from build123d import *

# Parameters (mm, degrees)
PAD_DEPTH = 1


with BuildPart() as part:
    # Sketch → Pad (new body)
    with BuildSketch(Plane.XY):
        with BuildLine():
            ThreePointArc((-1.225, 1.675), (-1.488415, 1.645732), (-1.73898, 1.559355))
            ThreePointArc((-4.225, 1), (-2.950915, 1.141565), (-1.73898, 1.559355))
            ThreePointArc((-4.225, 4), (-5.725, 2.5), (-4.225, 1))
            ThreePointArc((-4.225, 4), (-3.609451, 4.068394), (-3.023929, 4.270241))
            ThreePointArc((-1.225, 4.675), (-2.146951, 4.572561), (-3.023929, 4.270241))
            Line((-1.225, 4.675), (1.225012, 4.675))
            ThreePointArc((5.425, 0.475), (4.194853, 3.444844), (1.225012, 4.675))
            Line((5.425, -0.475), (5.425, 0.475))
            ThreePointArc((1.225, -4.675), (4.194848, -3.444848), (5.425, -0.475))
            Line((-1.225, -4.675), (1.225, -4.675))
            ThreePointArc((-3.023929, -4.270241), (-2.146951, -4.572561), (-1.225, -4.675))
            ThreePointArc((-3.023929, -4.270241), (-3.609451, -4.068394), (-4.225, -4))
            ThreePointArc((-4.225, -1), (-5.725, -2.5), (-4.225, -4))
            ThreePointArc((-1.73898, -1.559355), (-2.950915, -1.141565), (-4.225, -1))
            ThreePointArc((-1.73898, -1.559355), (-1.488415, -1.645732), (-1.225, -1.675))
            Line((-1.225, -1.675), (1.225, -1.675))
            ThreePointArc((1.225, -1.675), (2.073528, -1.323528), (2.425, -0.475))
            Line((2.425, 0.475), (2.425, -0.475))
            ThreePointArc((2.425, 0.475), (2.073532, 1.323524), (1.225012, 1.675))
            Line((-1.225, 1.675), (1.225012, 1.675))
        make_face()
    extrude(amount=PAD_DEPTH)


solid = part.part
Geometry check sheet. Reference: the model listing, model coordinates, mm. A direction names the side the tool comes from. Coordinates: 2 decimals unless noted, no trailing zeros. Order: outer loops, then holes, each group sorted by start corner. A loop starts at its lowest first (then second) coordinate and runs counter-clockwise, first axis right, second up. Notation, with made-up numbers: (54.25, -10) - (71.25, -10) arc R10 cw to (71.25, -5) - close; hole circle Ø8 at (0.5, 41.5). An arc over 180 degrees is marked (long way). Answer in a Markdown table with one row per item. Add a question column.
1) Gauge pin test, flat end, axial feed: P1, Ø1, axis at x = 0.5, y = 0.5, coming from the -Z side. Record the tip position at first contact, or that the pin passes through.
2) Cross-section at A-A, the plane x = 0. Record the cut outline in (y, z) (3 decimals), then the cut area to 3 significant figures.
3) Cross-section at C-C, the plane x = 1.5. Record the cut outline in (y, z).
4) Cross-section at B-B, the plane z = 0.6. Record the cut outline in (x, y) (3 decimals), then the cut area to 3 significant figures.
5) Set-up check for faces 4 (the flat face through (0, 2, 0)), 5 (the flat face through (0, -1.675, 0.5)), 6 (the flat face through (2.425, 0, 0.5)): record each of +Z, -Z, +X, -X, +Y, -Y from which the full face is reachable in a straight line by a thin tool's end or side.
6) Material ranges on line 1 along Y through (x, z) = (-4.25, 0.45); line 2 along Y through (x, z) = (1.25, 0.85); line 3 along X through (y, z) = (-0.25, 0.5) (3 decimals), recorded low to high. Write a range as [from, to].
7) Release check for a two-part mould opening along Y. For faces 1 (the cylindrical face through (-5.725, -2.467, 0.493)), 2 (the flat face through (0, -4.675, 0.5)), 3 (the flat face through (5.425, 0, 0.5)) record: +Y half, -Y half, draft (parallel to the pull), parting line (faces both ways), or undercut.
8) Cross-section at D-D, the plane y = 2.5. Record the cut outline in (x, z) (3 decimals).
Check result:
| question | item | result |
|---|---|---|
| 1 | P1 | passes through |
| 2 | outline | (-4.675, 0) - (-1.675, 0) - (-1.675, 1) - (-4.675, 1) - close; (1.675, 0) - (4.675, 0) - (4.675, 1) - (1.675, 1) - close |
| 2 | area | 6.00 mm² |
| 3 | outline | (-4.67, 0) - (-1.64, 0) - (-1.64, 1) - (-4.67, 1) - close; (1.64, 0) - (4.67, 0) - (4.67, 1) - (1.64, 1) - close |
| 4 | outline | (-4.225, -4) arc R2.804 cw to (-3.024, -4.27) arc R4.2 ccw to (-1.225, -4.675) - (1.225, -4.675) arc R4.2 ccw to (5.425, -0.475) - (5.425, 0.475) arc R4.2 ccw to (1.225, 4.675) - (-1.225, 4.675) arc R4.2 ccw to (-3.024, 4.27) arc R2.804 cw to (-4.225, 4) arc R1.5 ccw to (-4.225, 1) arc R5.804 ccw to (-1.739, 1.559) arc R1.2 cw to (-1.225, 1.675) - (1.225, 1.675) arc R1.2 cw to (2.425, 0.475) - (2.425, -0.475) arc R1.2 cw to (1.225, -1.675) - (-1.225, -1.675) arc R1.2 cw to (-1.739, -1.559) arc R5.804 ccw to (-4.225, -1) arc R1.5 ccw to start |
| 4 | area | 68.7 mm² |
| 5 | face 4 | -Z, +X, -X, +Y, -Y |
| 5 | face 5 | +Z, -Z |
| 5 | face 6 | +Z, -Z, -X |
| 6 | line 1 | y = [-4, -1], [1, 4] |
| 6 | line 2 | y = [-4.67, -1.67], [1.67, 4.67] |
| 6 | line 3 | x = [2.425, 5.425] |
| 7 | face 1 | undercut |
| 7 | face 2 | -Y half |
| 7 | face 3 | draft |
| 8 | outline | (-5.725, 0) - (4.905, 0) - (4.905, 1) - (-5.725, 1) - close |
